Verification items for the finished model (mm, model axes). Face numbers are marked on the shaded views. A direction names the side the tool comes from. Coordinates: 2 decimals unless noted, no trailing zeros. Order: outer loops, then holes, each group sorted by start corner. A loop starts at its lowest first (then second) coordinate and runs counter-clockwise, first axis right, second up. Notation, with made-up numbers: M 49,5.5 L 94,5.5 A18 cw 94,40.5 Z; hole C -8.5,51 d11. An arc over 180 degrees is marked long. Return JSON: item names as keys, results as strings.
Autodesk Inventor part; units mm, degrees
ref_plane "YZ Plane" through (0, 0, 0) normal (1, 0, 0) x (0, 1, 0)
ref_plane "XZ Plane" through (0, 0, 0) normal (0, 1, 0) x (-1, 0, 0)
ref_plane "XY Plane" through (0, 0, 0) normal (0, 0, 1) x (1, 0, 0)
sketch "Sketch1" plane through (0, 0, 0) normal (0, 0, 1) x (1, 0, 0)
  circle A0 centre (0, 0) radius 28.194
  dimension "d0" = 56.388
extrude "Extrusion1" add sketch "Sketch1" along normal blind 15.24
sketch "Sketch2" plane through (0, 0, 15.24) normal (0, 0, 1) x (1, 0, 0)
  circle A0 centre (0, 0) radius 28.194
  line L0 (0, 28.194) -> (19.1738, 28.194) construction
ref_plane "Work Plane1" through (0, 28.194, 15.24) normal (0, -1, 0) x (1, 0, 0)
sketch "Sketch3" plane through (0, 28.194, 15.24) normal (0, -1, 0) x (1, 0, 0)
  line L0 (-28.194, -15.24) -> (28.194, -15.24)
  line L1 (-28.194, -15.24) -> (37.5113, -11.7965)
  line L2 (-28.194, -15.24) -> (37.6014, -15.24) construction
  line L3 (37.5113, -11.7965) -> (37.5113, -25.6929)
  line L4 (37.5113, -25.6929) -> (-28.194, -15.24)
  point P0 (0, -15.24)
  dimension "d3" = 3
extrude "Extrusion2" cut sketch "Sketch3" along normal blind 152.4
sketch "Sketch4" plane through (0, 0, 1.4776) normal (0.052336, 0, -0.9986295) x (-0.9986295, 0, -0.052336)
  circle A0 centre (0.0773, 0) radius 35.814
  dimension "d6" = 71.628
extrude "Extrusion3" add sketch "Sketch4" along normal blind 2.54
properties part number "coilpiece2"
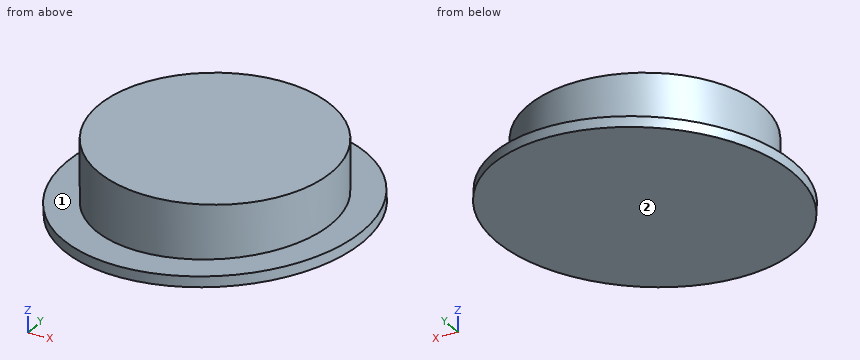
Q1. Go/stop test with flat-tipped pins: pin 1 (6 mm diameter, centred on x = -10, z = 1, fed in from +Y); pin 2 (6 mm diameter, centred on y = -8, z = 12.5, fed in from +X); pin 3 (4 mm diameter, centred on x = 7.5, z = 5.5, fed in from -Y). Record where each tip stops, or that it passes through.
Values:
{"pin 1": "y = 35.14", "pin 2": "x = 27.75", "pin 3": "y = -27.65"}
Q2. Cross-section at C-C, the plane y = 0. Record the boundary of the cut face in (x, z).
Values:
{"outline": "M -35.84,-0.4 L -35.71,-2.94 L 35.82,0.81 L 35.69,3.35 L 28.19,2.96 L 28.19,15.24 L -28.19,15.24 L -28.19,0 Z"}
Q3. Cross-section at A-A, the plane y = -15.5. Record the boundary of the cut face in (x, z), and give its area (3 significant figures).
Values:
{"outline": "M -32.32,-0.22 L -32.19,-2.75 L 32.3,0.63 L 32.16,3.16 L 23.55,2.71 L 23.55,15.24 L -23.55,15.24 L -23.55,0.24 Z", "area": "812 mm^2"}
Q4. Material ranges on line 1 along X through (y, z) = (-0.5, 13.5); line 2 along Z through (x, y) = (20, 22.5); line 3 along X through (y, z) = (24.5, 7.5), recorded low to high.
Values:
{"line 1": "-28.19 to 28.19", "line 2": "-0.02 to 2.53", "line 3": "-13.95 to 13.95"}
Q5. Cross-section at B-B, the plane z = 9.5. Record the boundary of the cut face in (x, y), and give its area (3 significant figures).
Values:
{"outline": "C 0,0 d56.39", "area": "2,500 mm^2"}
Q6. Tool access check on the marked faces 1 and 2. Record the directions out of +Z, -Z, +X, -X, +Y, -Y that give a thin tool (end or side, any length) a straight path to the whole face; none if there is none.
Values:
{"face 1": "+Z", "face 2": "-Z, +X, +Y, -Y"}
